from build123d import *

# Parameters (mm, degrees)
ESQUISSE1_W        = 300
ESQUISSE1_H        = 300
BOSS_EXTRU_1_DEPTH = 5
ESQUISSE2_R        = 4
BOSS_EXTRU_2_DEPTH = 300
BOSS_EXTRU_4_DEPTH = 50


with BuildPart() as part:
    # Esquisse1 → Boss.-Extru.1 (new body)
    with BuildSketch(Plane.XY):
        with Locations((150, -150)):
            Rectangle(ESQUISSE1_W, ESQUISSE1_H)
    extrude(amount=BOSS_EXTRU_1_DEPTH)

    # Esquisse2 → Boss.-Extru.2 (add)
    with BuildSketch(Plane.XY.offset(5)):
        with Locations((15, -70)):
            Circle(ESQUISSE2_R)
        with Locations((285, -70)):
            Circle(ESQUISSE2_R)
    extrude(amount=BOSS_EXTRU_2_DEPTH)

    # Esquisse5 → Boss.-Extru.4 (add)
    with BuildSketch(Plane.XY.offset(5)):
        with BuildLine():
            ThreePointArc((95, -122.991547009), (150, -148.920572223), (205, -122.991547009))
            ThreePointArc((205, -122.991547009), (207.11161857, -122.788897028), (207.314268551, -124.900515598))
            ThreePointArc((207.314268551, -124.900515598), (150, -151.920572223), (92.685731449, -124.900515598))
            ThreePointArc((92.685731449, -124.900515598), (92.88838143, -122.788897028), (95, -122.991547009))
        make_face()
    extrude(amount=BOSS_EXTRU_4_DEPTH)


solid = part.part
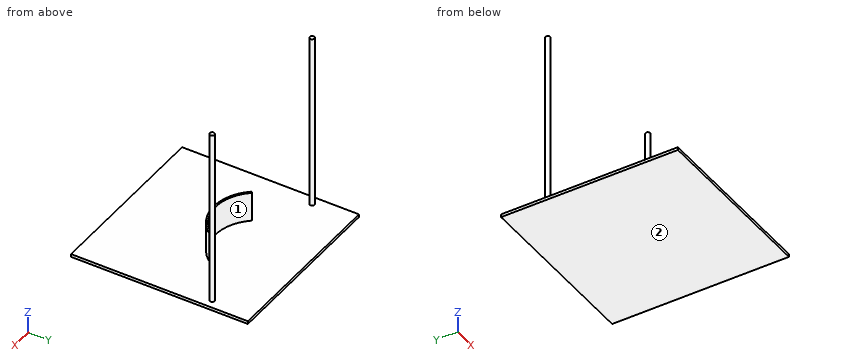
Model file for the job. Use its own axes, mm. Face numbers are marked on the shaded views. Give positions to 0.01 mm unless a question says otherwise; leave off trailing zeros. Order: outer loops, then holes, each group sorted by start corner. A loop starts at its lowest first (then second) coordinate and runs counter-clockwise, first axis right, second up. Notation, with made-up numbers: (0.5, 45.5) - (57.5, 45.5) arc R21 cw to (57.5, 74.5) - close; hole circle Ø7 at (56, 72.5). An arc over 180 degrees is marked (long way). Write item = value, one per line. Start each with the question number.
1. Two-plate mould, pull along X, no slides. Class the marked faces 1 and 2: pulls with the +X half, pulls with the -X half, needs draft (parallel to the pull), parting line crosses it, or undercut.
2. Probe line 1 along Z through (x, y) = (138, -91.5). List the from-to ranges inside material, lowest first.
3. Cut at C-C, the plane y = -248. List the corners of the cut face in (x, z).
4. Drop a flat-ended pin along its axis: P1, Ø6, axis at x = 145, y = -125, coming from the +Z side. Give the stop position or say it passes through.
5. Cut at B-B, the plane x = 140. List the corners of the cut face in (y, z), and give its area (3 significant figures).
6. Cut at D-D, the plane x = 212. List the corners of the cut face in (y, z), and give its area (3 significant figures).
7. Cut at A-A, the plane z = 184. List the corners of the cut face in (x, y), and give its area (3 significant figures).
Taken from the geometry:
q1.face_1 = undercut
q1.face_2 = needs draft
q2.line_1 = 0 to 5
q3.outline = (0, 0) - (300, 0) - (300, 5) - (0, 5) - close
q4.P1 = 5
q5.outline = (-300, 0) - (0, 0) - (0, 5) - (-148.22, 5) - (-148.22, 55) - (-151.24, 55) - (-151.24, 5) - (-300, 5) - close
q5.area = 1,650 mm²
q6.outline = (-300, 0) - (0, 0) - (0, 5) - (-300, 5) - close
q6.area = 1,500 mm²
q7.outline = circle Ø8 at (15, -70); circle Ø8 at (285, -70)
q7.area = 101 mm²
